For this review, use the dimensioned drawing (mm, ordinates from the lowest corner) and the shaded views. A direction names the side the tool comes from. Coordinates: 2 decimals unless noted, no trailing zeros. Write each loop counter-clockwise with the first axis right and the second up, starting at its lowest first coordinate (ties: lowest second). Pieces come first, ordered by that corner, then holes. Notation, with made-up numbers: M -34,15.5 L -1,15.5 A23 cw -1,47.5 Z; hole C 68.5,54 d8. An arc over 180 degrees is marked long. One line per question, with ' | ' between items.
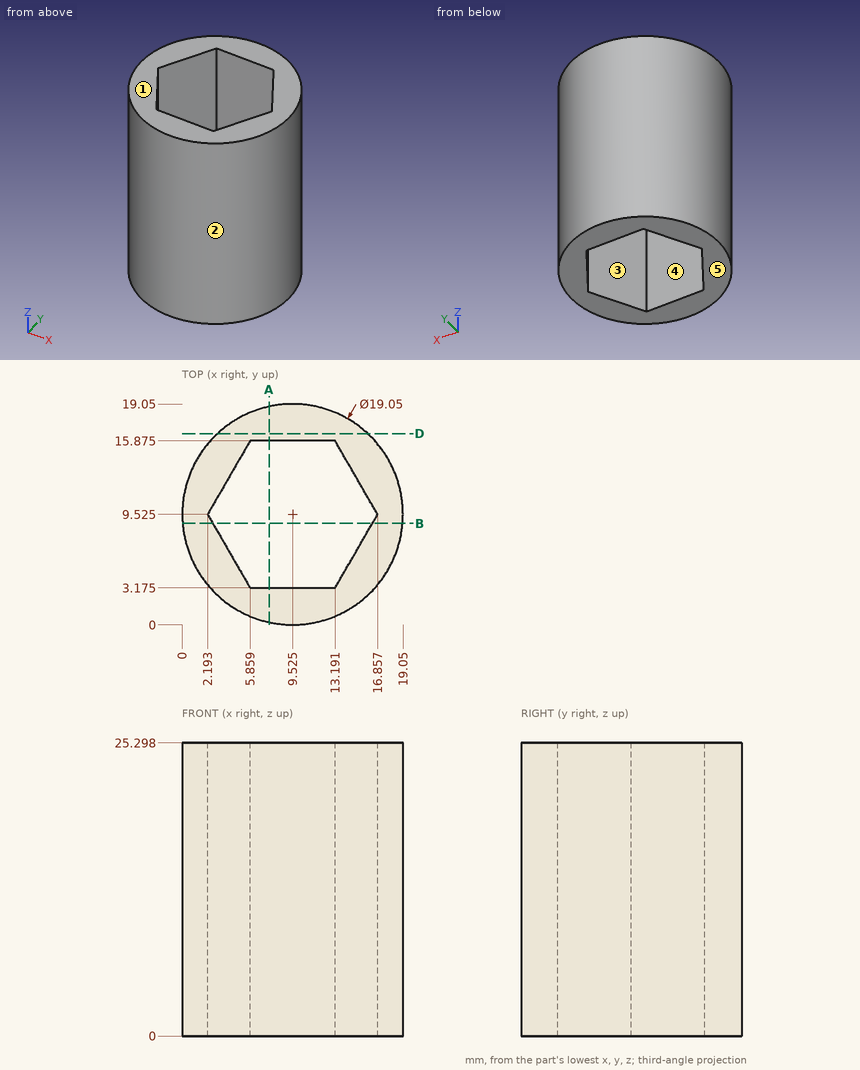
1. Take a section at A-A (x = 7.5). Write out the cut boundary in (y, z) (1 decimal).
Answer sheet:
outline: M 0.2,0 L 3.2,0 L 3.2,25.3 L 0.2,25.3 Z; M 15.9,0 L 18.8,0 L 18.8,25.3 L 15.9,25.3 Z
2. Draft analysis for pull direction Y (two halves, no side actions). For the marked faces 1, 2 and 3, state which applies: pulls with the +Y half, pulls with the -Y half, needs draft (parallel to the pull), parting line crosses it, or undercut.
Answer sheet:
face 1: needs draft | face 2: parting line crosses it | face 3: undercut
3. Insertion check: pin 1 Ø2 at (x, z) = (11.5, 9) entering from +Y; pin 2 Ø5 at (y, z) = (14, 7) entering from +X. Each pin has a flat end and moves straight along its axis. Give the tip position at first contact, or say it passes through.
Answer sheet:
pin 1: y = 19 | pin 2: x = 18.84
4. Tool access review of the marked faces 4 and 5: name each direction out of +Z, -Z, +X, -X, +Y, -Y from which nothing blocks a thin tool from reaching the whole face with its end or side.
Answer sheet:
face 4: +Z, -Z | face 5: -Z, +X, -X, +Y, -Y
5. To check wall thickness, follow line 1 along Y through (x, z) = (9.75, 9.25) (1 decimal); line 2 along X through (y, z) = (14.25, 20) (1 decimal); line 3 along Y through (x, z) = (12, 13) (1 decimal). State the ranges of each line that lie inside material, in increasing order. Write a range as [from, to].
Answer sheet:
line 1: [0, 3.2], [15.9, 19] | line 2: [1.3, 4.9], [14.1, 17.8] | line 3: [0.3, 3.2], [15.9, 18.7]
6. Take a section at B-B (y = 8.75). Write out the cut boundary in (x, z), then the cut area to 3 significant figures.
Answer sheet:
outline: M 0.03,0 L 2.64,0 L 2.64,25.3 L 0.03,25.3 Z; M 16.41,0 L 19.02,0 L 19.02,25.3 L 16.41,25.3 Z | area: 132 mm^2
7. Take a section at D-D (y = 16.5). Write out the cut boundary in (x, z), then the cut area to 3 significant figures.
Answer sheet:
outline: M 3.04,0 L 16.01,0 L 16.01,25.3 L 3.04,25.3 Z | area: 328 mm^2
